from build123d import *

# Parameters (mm, degrees)
F0_W     = 50
F0_H     = 100
F1_DEPTH = 20
F2_R     = 6
F3_DEPTH = 25
F4_R     = 20
F5_R     = 20
F6_W     = 37
F6_H     = 12.5
F7_DEPTH = 50.001
F8_R     = 3.5
F9_DEPTH = 20.001


with BuildPart() as f1:
    # F0 (on Top) → F1 (new body)
    with BuildSketch(Plane.XY):
        with Locations((6.21234, -33.364211)):
            Rectangle(F0_W, F0_H)
    extrude(amount=F1_DEPTH)

    # F2 (on face) → F3 (cut)
    with BuildSketch(Plane.XY.offset(20)):
        with Locations((6.21234, 4.635789)):
            Circle(F2_R)
    extrude(amount=-F3_DEPTH, mode=Mode.SUBTRACT)

    # F4
    f4_edges = [f1.edges().sort_by_distance(p)[0] for p in [
        (31.21234, 16.635789, 10),
    ]]
    fillet(f4_edges, radius=F4_R)

    # F5
    f5_edges = [f1.edges().sort_by_distance(p)[0] for p in [
        (-18.78766, 16.635789, 10),
    ]]
    fillet(f5_edges, radius=F5_R)

    # F6 (on face) → F7 (cut, through all)
    with BuildSketch(Plane.YZ.offset(31.21234)):
        with Locations((-49.864211, 13.75)):
            Rectangle(F6_W, F6_H)
    extrude(amount=-F7_DEPTH, mode=Mode.SUBTRACT)

    # F8 (on face) → F9 (cut, through all)
    with BuildSketch(Plane(origin=(0, 0, 0), x_dir=(1, 0, 0), z_dir=(0, 0, -1))):
        with Locations((6.21234, 51.364211)):
            Circle(F8_R)
        with Locations((6.21234, 21.364211)):
            Circle(F8_R)
        with Locations((6.21234, 76.364211)):
            Circle(F8_R)
    extrude(amount=-F9_DEPTH, mode=Mode.SUBTRACT)


solid = f1.part
The model under review builds one solid part; all positions refer to its coordinate system, in mm. A direction names the side the tool comes from. Coordinates: 2 decimals unless noted, no trailing zeros. Loops run counter-clockwise (first coordinate to the right, second up) from the corner with the lowest first, then second, coordinate; pieces in that order, holes last. Notation, with made-up numbers: (68.25, 75) -> (108.25, 75) arc R13 ccw to (108.25, 96) -> close; hole circle Ø8 at (25.5, 48). An arc over 180 degrees is marked (long way). Use a Markdown table: item, result. Add a question column.
1. Machinability: for faces 5 (the face through (7, -68.364, 14)), 6 (the face through (6, -7, 20)), which of the approach directions +Z, -Z, +X, -X, +Y, -Y give a long, thin tool a straight path to every point of the face, cutting with its end or side? Answer none if there is none.
2. Add section B-B on y = 6. Write out the cut boundary in (x, z).
3. Clearance check with flat-ended pins moving along their axes: pin 1 Ø5.5 at (x, y) = (6.21, -51.36) entering from +Z; pin 2 Ø1.5 at (y, z) = (1, 12) entering from -X; pin 3 Ø11 at (x, y) = (15.5, -56) entering from +Z. State where each tip first meets the part, or that it passes through.
4. Add section C-C on z = 5.75. Write out the cut boundary in (x, y), plus the area to 3 significant figures.
5. Draft analysis for pull direction Y (two halves, no side actions). For faces 1 (the face through (25.2, 10.93, 10.14)), 2 (the face through (0.22, 4.9, 10.14)), 3 (the face through (7, -46, 7.5)), 4 (the face through (6, -72, 20)), state which applies: pulls with the +Y half, pulls with the -Y half, needs draft (parallel to the pull), parting line crosses it, or undercut.
6. To check wall thickness, follow line 1 (Y direction, x = 6.5, z = 8.25); line 2 (Y direction, x = 9, z = 3.75); line 3 (Y direction, x = 11.5, z = 13.5). State the ranges of each line that lie inside material, in increasing order.
7. Add section A-A on z = 17.25. Write out the cut boundary in (x, y).
8. Add section D-D on x = 23. Write out the cut boundary in (y, z).
Returned:
| question | item | result |
|---|---|---|
| 1 | face 5 | +Z, +X, -X |
| 1 | face 6 | +Z, +X, -X, +Y, -Y |
| 2 | outline | (-16.46, 0) -> (0.37, 0) -> (0.37, 20) -> (-16.46, 20) -> close; (12.06, 0) -> (28.88, 0) -> (28.88, 20) -> (12.06, 20) -> close |
| 3 | pin 1 | passes through |
| 3 | pin 2 | stops at x = -18.46 |
| 3 | pin 3 | stops at z = 7.5 |
| 4 | outline | (-18.79, -83.36) -> (31.21, -83.36) -> (31.21, -3.36) arc R20 ccw to (11.21, 16.64) -> (1.21, 16.64) arc R20 ccw to (-18.79, -3.36) -> close; hole circle Ø12 at (6.21, 4.64); hole circle Ø7 at (6.21, -76.36); hole circle Ø7 at (6.21, -51.36); hole circle Ø7 at (6.21, -21.36) |
| 4 | area | 4,600 mm² |
| 5 | face 1 | pulls with the +Y half |
| 5 | face 2 | undercut |
| 5 | face 3 | undercut |
| 5 | face 4 | needs draft |
| 6 | line 1 | y = -83.36 to -79.85, -72.88 to -68.36, -31.36 to -24.85, -17.88 to -1.36, 10.63 to 16.64 |
| 6 | line 2 | y = -83.36 to -78.48, -74.25 to -53.48, -49.25 to -23.48, -19.25 to -0.68, 9.95 to 16.64 |
| 6 | line 3 | y = -83.36 to -68.36, -31.36 to 1.8, 7.47 to 16.63 |
| 7 | outline | (-18.79, -83.36) -> (31.21, -83.36) -> (31.21, -68.36) -> (-18.79, -68.36) -> close; (-18.79, -31.36) -> (31.21, -31.36) -> (31.21, -3.36) arc R20 ccw to (11.21, 16.64) -> (1.21, 16.64) arc R20 ccw to (-18.79, -3.36) -> close; hole circle Ø12 at (6.21, 4.64); hole circle Ø7 at (6.21, -76.36); hole circle Ø7 at (6.21, -21.36) |
| 8 | outline | (-83.36, 0) -> (12.79, 0) -> (12.79, 20) -> (-31.36, 20) -> (-31.36, 7.5) -> (-68.36, 7.5) -> (-68.36, 20) -> (-83.36, 20) -> close |
